Here's how the part is built. I have some questions about the finished solid (model axes, mm). A direction names the side the tool comes from. Coordinates: 2 decimals unless noted, no trailing zeros. Loops run counter-clockwise (first coordinate to the right, second up) from the corner with the lowest first, then second, coordinate; pieces in that order, holes last.
Autodesk Inventor part; units mm, degrees
ref_plane "YZ Plane" through (0, 0, 0) normal (1, 0, 0) x (0, 1, 0)
ref_plane "XZ Plane" through (0, 0, 0) normal (0, 1, 0) x (-1, 0, 0)
ref_plane "XY Plane" through (0, 0, 0) normal (0, 0, 1) x (1, 0, 0)
sketch "Sketch1" plane through (0, 0, 0) normal (0, 0, 1) x (1, 0, 0)
  circle A0 centre (0, 0) radius 5.175
  dimension "d0" = 10.35
extrude "Extrusion1" add sketch "Sketch1" along normal blind 6.75
sketch "Sketch2" plane through (0, 0, 6.75) normal (0, 0, 1) x (1, 0, 0)
  circle A0 centre (0, 0) radius 5.375
  dimension "d3" = 10.75
extrude "Extrusion2" add sketch "Sketch2" along normal blind 15.5
sketch "Sketch3" plane through (0, 0, 22.25) normal (0, 0, 1) x (1, 0, 0)
  circle A0 centre (0, 0) radius 9.05
  dimension "d6" = 18.1
extrude "Extrusion3" add sketch "Sketch3" along normal blind 6.5
chamfer "Chamfer1" distance 6.5 angle 15 1 edges at (-9.05, 0, 28.75) measured on face at (8.9328, -1.4517, 26.5833)
sketch "Sketch4" plane through (0, 0, 0) normal (0, 0, -1) x (-1, 0, 0)
  circle A0 centre (0, 0) radius 5.175
  line L0 (2.55, 1.5) -> (2.05, 1.5)
  line L1 (2.05, 1.5) -> (2.05, -1.5)
  line L2 (2.05, -1.5) -> (2.55, -1.5)
  line L3 (2.55, -1.5) -> (2.55, 1.5)
  line L4 (-2.05, 1.5) -> (-2.55, 1.5)
  line L5 (-2.55, 1.5) -> (-2.55, -1.5)
  line L6 (-2.55, -1.5) -> (-2.05, -1.5)
  line L7 (-2.05, -1.5) -> (-2.05, 1.5)
  dimension "d12" = 0.5
  dimension "d13" = 3
  dimension "d14" = 0.5
  dimension "d15" = 3
  dimension "d16" = 5.1
  dimension "d17" = 2.625
  dimension "d18" = 2.625
  dimension "d19" = 3.675
  dimension "d20" = 3.675
extrude "Extrusion4" add sketch "Sketch4" along normal blind 6 contours L3 L2 L1 L0 | L7 L6 L5 L4
fillet "Fillet1" radius 1.5 4 edges at (-2.3, 1.5, -6) (-2.3, -1.5, -6) (2.3, 1.5, -6) (2.3, -1.5, -6)
sketch "Sketch5" plane through (-2.55, -1.5, 0) normal (-1, 0, 0) x (0, 0, 1)
  line L0 (-4.7053, 1.5) -> (-3.2606, 1.5) construction
  line L1 (-4.7053, 0.9641) -> (-3.2606, 0.9641)
  line L2 (-3.2606, 2.0359) -> (-4.7053, 2.0359)
  arc A0 (-4.7053, 2.0359) -> (-4.7053, 0.9641) centre (-4.7053, 1.5) ccw
  arc A1 (-3.2606, 0.9641) -> (-3.2606, 2.0359) centre (-3.2606, 1.5) ccw
  line L3 (0, 0) -> (-4.5, 0)
  line L4 (0, 3) -> (-4.5, 3)
  point P0 (0, 1.5)
  point P1 (-3.983, 1.5)
  dimension "d24" = 1.5
  dimension "d25" = 1.5
extrude "Extrusion5" cut sketch "Sketch5" against normal through all
sketch "Sketch6" plane through (0, 0, 28.75) normal (0, 0, 1) x (1, 0, 0)
  circle A0 centre (0, 0) radius 6
  dimension "d28" = 12
extrude "Extrusion6" add sketch "Sketch6" along normal blind 4.5
equation "\"d17\" = d18"
equation "\"d19\" = d20"
equation "\"d24\" = d25"
properties part number "przycisk"
Q1. We'd pull the mould along X, two halves only. Please class faces 1 (the flat face through (2.05, 0, -2)), 2 (the flat face through (0, 0, 33.25)), 3 (the flat face through (2.55, 0, -2)): pulls with the +X half, pulls with the -X half, needs draft (parallel to the pull), parting line crosses it, or undercut.
Q2. For faces 4 (the cylindrical face through (-6, 0, 31)), 5 (the flat face through (-2.55, 0, -2)), 6 (the flat face through (4, -4, 22.25)), 7 (the flat face through (-2.05, 0, -2)), which set-ups out of +Z, -Z, +X, -X, +Y, -Y let a thin tool reach every point of the face, with its end or its side?
Q3. Suppose I cut it at B-B on z = 15. Write out the boundary of the cut face in (x, y) (3 decimals).
Q4. Suppose I cut it at C-C on z = 24.5. Write out the boundary of the cut face in (x, y).
Q5. Will these pins go through, and if not, where does the flat tip stop? P1, Ø0.9, axis at y = -0.5, z = -2.5, coming from the -X side; P2, Ø10, axis at x = 1.5, z = 16, coming from the +Y side (3 decimals); P3, Ø0.9, axis at y = 0.5, z = -4, coming from the +X side.
Q6. Please list where these lines run through material, in increasing order: probe 1 along Y at (x, z) = (-0.25, 8); probe 2 along Z at (x, y) = (-4, 5.5); probe 3 along Z at (x, y) = (-1.5, -3).
Check values:
1. face 1: undercut
1. face 2: needs draft
1. face 3: pulls with the +X half
2. face 4: +Z
2. face 5: -Z, -X, +Y, -Y
2. face 6: -Z
2. face 7: -Z, +Y, -Y
3. outline: circle Ø10.75 at (0, 0)
4. outline: circle Ø16.89 at (0, 0)
5. P1: stops at x = -2.55
5. P2: stops at y = 5.375
5. P3: stops at x = 2.55
6. probe 1: y = -5.37 to 5.37
6. probe 2: z = 22.25 to 28.75
6. probe 3: z = 0 to 33.25
